Answer from the drawing. Dimensions are ordinates in mm from the lowest x, y and z of the part. Give positions to 0.01 mm unless a question says otherwise; leave off trailing zeros.
(1) Each of these flat-tipped pins is pushed along its axis until it touches: P1, Ø2, axis at y = 22, z = 11.5, coming from the -X side; P2, Ø3, axis at x = 12, z = 14.5, coming from the +Y side; P3, Ø2, axis at x = 15.5, z = 16.5, coming from the +Y side; P4, Ø6, axis at x = 8, z = 13, coming from the -Y side. Where does it stop, or does it pass through?
(2) Determine the mould class of the marked faces 1, 2 and 3 for opening direction X: pulls with the +X half, pulls with the -X half, needs draft (parallel to the pull), parting line crosses it, or undercut.
(3) Straight lines are drawn through the part: probe 1 along X at (y, z) = (16, 13.5); probe 2 along X at (y, z) = (26.5, 11); probe 3 along Y at (x, z) = (25, 11.75). For each, find the intervals that lie inside material, in ascending order.
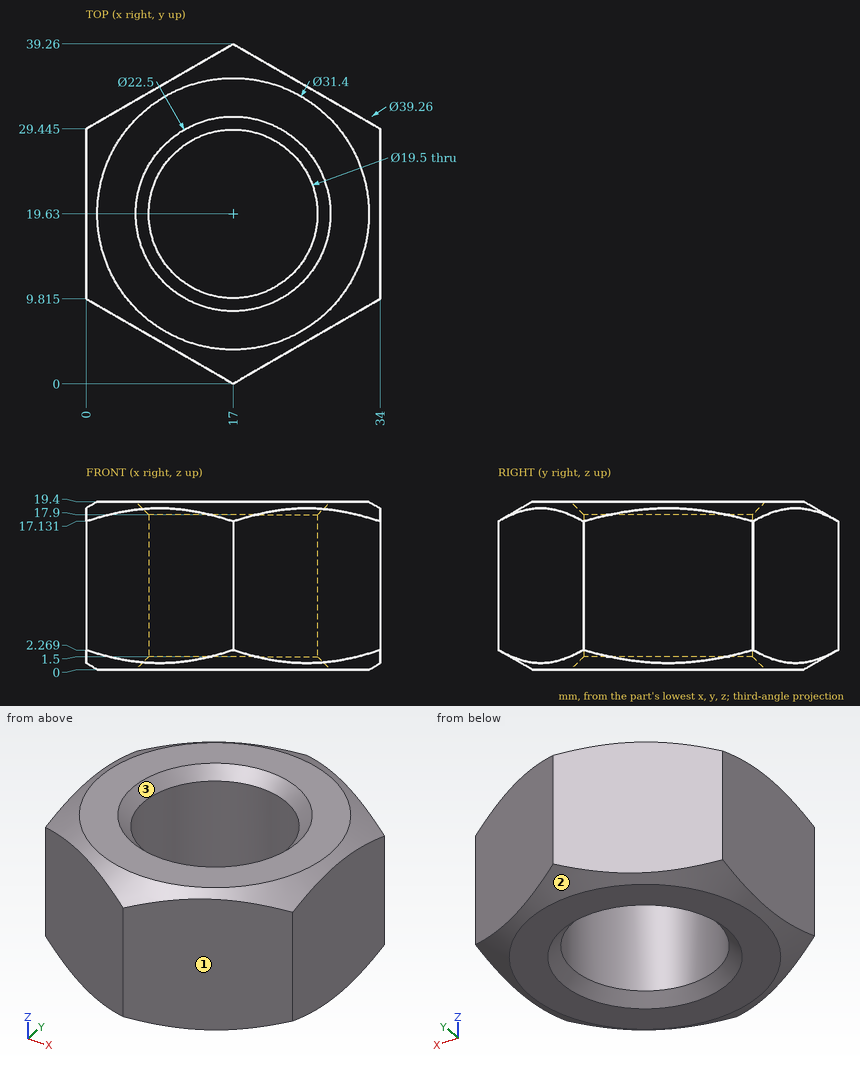
Entries:
1. P1: stops at x = 0
1. P2: stops at y = 37.24
1. P3: stops at y = 38.97
1. P4: stops at y = 3.46
2. face 1: pulls with the +X half
2. face 2: parting line crosses it
2. face 3: undercut
3. probe 1: x = 0 to 7.95, 26.05 to 34
3. probe 2: x = 0 to 10.08, 23.92 to 34
3. probe 3: y = 4.62 to 14.06, 25.2 to 34.64
